```python
from build123d import *

# Parameters (mm, degrees)
PAD_DEPTH       = 2.5
SKETCH002_R     = 1.6
SKETCH002_R_2   = 1.45
POCKET001_DEPTH = 4.001
SKETCH003_R     = 2.5
SKETCH003_R_2   = 1.45
SKETCH003_R_3   = 1.6
PAD001_DEPTH    = 1.25


with BuildPart() as part:
    # Sketch → Pad (new body, symmetric)
    with BuildSketch(Plane.XZ):
        Polygon((-27.15, 0), (27.15, 0), (32.15, 0), (32.15, -4), (-32.15, -4), (-32.15, 0), align=None)
    extrude(amount=PAD_DEPTH, both=True)

    # Sketch002 → Pocket001 (cut, through all)
    with BuildSketch(Plane.XY):
        with Locations((29.65, 0)):
            Circle(SKETCH002_R)
        with Locations((10.65, 0)):
            Circle(SKETCH002_R_2)
        with Locations((-29.65, 0)):
            Circle(SKETCH002_R)
    extrude(amount=-POCKET001_DEPTH, mode=Mode.SUBTRACT)

    # Sketch003 → Pad001 (join)
    with BuildSketch(Plane.XY):
        with Locations((10.65, 0)):
            Circle(SKETCH003_R)
        with Locations((10.65, 0)):
            Circle(SKETCH003_R_2, mode=Mode.SUBTRACT)
        with Locations((29.65, 0)):
            Circle(SKETCH003_R)
        with Locations((29.65, 0)):
            Circle(SKETCH003_R_3, mode=Mode.SUBTRACT)
    extrude(amount=PAD001_DEPTH)


solid = part.part
```
Could you check a few things on this model? Use its own coordinates, in mm. A direction names the side the tool comes from. Round coordinates to 2 decimals unless told otherwise and drop trailing zeros. Loops run counter-clockwise (first coordinate to the right, second up) from the corner with the lowest first, then second, coordinate; pieces in that order, holes last.
Q1. I want a section at D-D (z = 0.65). Write out the boundary of the cut face in (x, y).
Q2. I want a section at C-C (y = -0.6). Write out the boundary of the cut face in (x, z), and give its area (3 significant figures).
Q3. I want a section at B-B (z = -2.7). Write out the boundary of the cut face in (x, y), and give its area (3 significant figures).
Q4. Please list where these lines run through material, in increasing order: L1, parallel to X at y = -0.1, z = -0.7; L2, parallel to Y at x = 10.65, z = -3.1; L3, parallel to X at y = -1.1, z = -1.1.
Q5. Thinking about a two-plate mould opening in Y: for faces 1 (the flat face through (0, -2.5, -2)), 2 (the cylindrical face through (-31.25, 0.07, -1.97)), 3 (the cylindrical face through (8.666, -1.521, 0.616)), 4 (the flat face through (12, -1, 1.25)), which applies, pulls with the +Y half, pulls with the -Y half, needs draft (parallel to the pull), parting line crosses it, or undercut?
Q6. I want a section at A-A (x = -29.65). Write out the boundary of the cut face in (y, z).
Q7. On a 3-axis mill with a long thin cutter (end or side, diameter ignored), from which of +Z, -Z, +X, -X, +Y, -Y can I reach the whole of each face in a straight line? I mean faces 5 (the cylindrical face through (31.96, -0.96, 0.62)), 6 (the flat face through (31.6, 1.9, 0)), 7 (the flat face through (31.6, -1.9, 0)). Say none if no direction works.
Q8. For P1, Ø1.9, axis at x = -29.65, y = 0, coming from the +Z side, with a flat end and sliding along its axis, tell me the tip position at first contact or that it passes through.
Answer below:
1. outline: circle Ø5 at (10.65, 0); circle Ø5 at (29.65, 0); hole circle Ø2.9 at (10.65, 0); hole circle Ø3.2 at (29.65, 0)
2. outline: (-32.15, -4) - (-31.13, -4) - (-31.13, 0) - (-32.15, 0) - close; (-28.17, -4) - (9.33, -4) - (9.33, 1.25) - (8.22, 1.25) - (8.22, 0) - (-28.17, 0) - close; (11.97, -4) - (28.17, -4) - (28.17, 1.25) - (27.22, 1.25) - (27.22, 0) - (13.08, 0) - (13.08, 1.25) - (11.97, 1.25) - close; (31.13, -4) - (32.15, -4) - (32.15, 0) - (32.08, 0) - (32.08, 1.25) - (31.13, 1.25) - close
2. area: 228 mm2
3. outline: (-32.15, -2.5) - (32.15, -2.5) - (32.15, 2.5) - (-32.15, 2.5) - close; hole circle Ø3.2 at (-29.65, 0); hole circle Ø2.9 at (10.65, 0); hole circle Ø3.2 at (29.65, 0)
3. area: 299 mm2
4. L1: x = -32.15 to -31.25, -28.05 to 9.2, 12.1 to 28.05, 31.25 to 32.15
4. L2: y = -2.5 to -1.45, 1.45 to 2.5
4. L3: x = -32.15 to -30.81, -28.49 to 9.71, 11.59 to 28.49, 30.81 to 32.15
5. face 1: pulls with the -Y half
5. face 2: undercut
5. face 3: parting line crosses it
5. face 4: needs draft
6. outline: (-2.5, -4) - (-1.6, -4) - (-1.6, 0) - (-2.5, 0) - close; (1.6, -4) - (2.5, -4) - (2.5, 0) - (1.6, 0) - close
7. face 5: +Z
7. face 6: +Z, +X, +Y
7. face 7: +Z, +X, -Y
8. P1: passes through
